Autodesk Inventor part; units mm, degrees
ref_plane "YZ Plane" through (0, 0, 0) normal (1, 0, 0) x (0, 1, 0)
ref_plane "XZ Plane" through (0, 0, 0) normal (0, 1, 0) x (-1, 0, 0)
ref_plane "XY Plane" through (0, 0, 0) normal (0, 0, 1) x (1, 0, 0)
sketch "Sketch1" plane through (0, 0, 0) normal (0, 0, 1) x (1, 0, 0)
  arc A0 (0, 550) -> (-550, 0) centre (0, 0) ccw
  arc A1 (0, 450) -> (-450, 0) centre (0, 0) ccw
  line L0 (0, 550) -> (0, 450)
  line L1 (-450, 0) -> (-550, 0)
  point P0 (-500, 0)
  point P1 (0, 500)
  dimension "d0" = 1100
  dimension "d1" = 900
extrude "Plate1" add sketch "Sketch1" against normal blind 3
sketch "Sketch2" plane through (0, 0, 0) normal (0, 0, 1) x (1, 0, 0)
  line L0 (-550, 0) -> (-450, 0)
  arc A0 (0, 550) -> (-550, 0) centre (0, 0) ccw
  circle A1 centre (-461.9398, 191.3417) radius 5
  arc A2 (0, 450) -> (-450, 0) centre (0, 0) ccw
  line L1 (-415.7458, 172.2075) -> (-508.1337, 210.4759) construction
  point P0 (-461.9398, 191.3417)
  dimension "d4" = 10
  dimension "d5" = 22.5
extrude "Cut1" cut sketch "Sketch2" against normal through all
pattern_circular "Circular Pattern1" count 2 over 45 about axis through (0, 0, 0) along (0, 0, -1) of "Cut1"
equation "\"d0\" = Диаметр_вн"
equation "\"d1\" = d0 - 2 * Ширина_кольца"
equation "\"d4\" = Диаметр_отв"
equation "\"d6\" = Thickness"
equation "\"d2\" = Thickness"
equation "\"BendReliefWidth\" = Thickness"
equation "\"BendReliefDepth\" = 0.5 * Thickness"
equation "\"CornerReliefSize\" = 4 * Thickness"
equation "\"MinimumRemnant\" = 2 * Thickness"
equation "\"TransitionRadius\" = BendRadius"
equation "\"JacobiRadiusSize\" = BendRadius"
equation "\"GapSize\" = Thickness"
properties part number "BSH 501 segment" material "Stainless Steel"
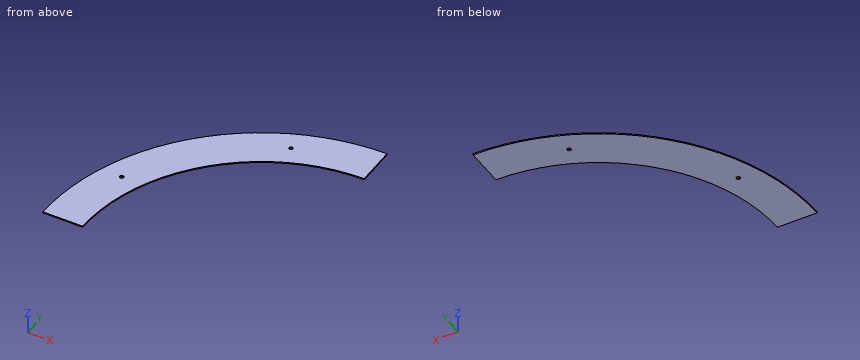
Read the model definition and answer for the solid it produces. Units are mm, in the model's axes. Coordinates: 2 decimals unless noted, no trailing zeros. Write each loop counter-clockwise with the first axis right and the second up, starting at its lowest first coordinate (ties: lowest second). Pieces come first, ordered by that corner, then holes. Notation, with made-up numbers: (59, 80.25) -> (70, 80.25) arc R12 cw to (70, 98.25) -> close; hole circle Ø5 at (5.5, 16). An arc over 180 degrees is marked (long way). Write item = value, one per line.
(1) Section B-B on x = -329 is taken. Write down the section's boundary in (y, z), plus the area to 3 significant figures.
From the geometry:
outline = (307.02, -3) -> (440.75, -3) -> (440.75, 0) -> (307.02, 0) -> close
area = 401 mm2
(2) Section C-C on y = 313 is taken. Write down the section's boundary in (x, z).
From the geometry:
outline = (-452.25, -3) -> (-323.31, -3) -> (-323.31, 0) -> (-452.25, 0) -> close
(3) Straight lines are drawn through the part: L1, parallel to Y at x = -90.5, z = -0.25; L2, parallel to Y at x = -330, z = -1.4; L3, parallel to X at y = 71, z = -1.25. For each, find the intervals that lie inside material, in ascending order. Write a range as from..to.
From the geometry:
L1 = 440.81..542.5
L2 = 305.94..440
L3 = -545.4..-444.36
(4) Given pin 1 Ø6 at (x, y) = (-461.94, 191.34) entering from +Z, flat-ended and moving along its own axis, determine where the tip first touches the part or whether it passes through.
From the geometry:
pin_1 = through
